Design review of the part shown in the three views and the two pictorial views. Dimensions are in mm from the part's minimum x, y and z. Coordinates: 2 decimals unless noted, no trailing zeros. Order: outer loops, then holes, each group sorted by start corner. A loop starts at its lowest first (then second) coordinate and runs counter-clockwise, first axis right, second up. Notation, with made-up numbers: (-5, 81) -> (48, 81) arc R24 ccw to (48, 120) -> close; hole circle Ø5 at (5.25, 64.25). An arc over 180 degrees is marked (long way). Write item = value, one per line. Start each with the question number.
1) Draft analysis for pull direction Z (two halves, no side actions). For the marked faces 1, 2 and 3, state which applies: +Z half, -Z half, draft (parallel to the pull), parting line (faces both ways), or undercut.
2) Insertion check: pin 1 Ø8 at (x, z) = (19.05, 12.7) entering from +Y. The pin has a flat end and moves straight along its axis. Give the tip position at first contact, or say it passes through.
3) Wall thickness on probe 1 along X at (y, z) = (6.35, 5.5); probe 2 along Y at (x, z) = (44.45, 11.5); probe 3 along Z at (x, y) = (31.75, 3.5): over which ranges is each line inside the solid? List them lowest first. Write a range as [from, to].
4) Consider section C-C on x = 19.05. Give the boundary of the cut face in (y, z), and give its area (3 significant figures).
5) Consider section B-B on z = 12.7. State how many separate pieces and enclosed holes the cut face has.
6) Consider section A-A on y = 6.35. Give the boundary of the cut face in (x, z), and give its area (3 significant figures).
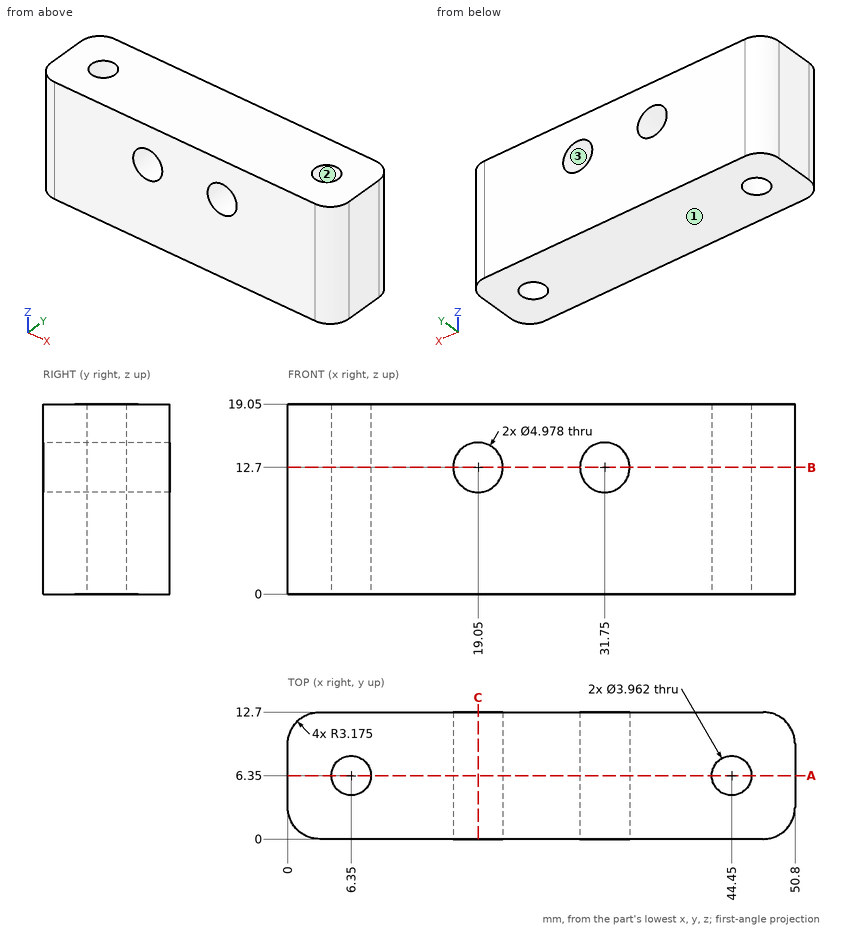
Answer sheet:
q1.face_1 = -Z half
q1.face_2 = draft
q1.face_3 = undercut
q2.pin_1 = 12.7
q3.probe_1 = [0, 4.37], [8.33, 42.47], [46.43, 50.8]
q3.probe_2 = [0, 4.37], [8.33, 12.7]
q3.probe_3 = [0, 10.21], [15.19, 19.05]
q4.outline = (0, 0) -> (12.7, 0) -> (12.7, 10.21) -> (0, 10.21) -> close; (0, 15.19) -> (12.7, 15.19) -> (12.7, 19.05) -> (0, 19.05) -> close
q4.area = 179 mm2
q5.separate_pieces = 3
q5.enclosed_holes = 2
q6.outline = (0, 0) -> (4.37, 0) -> (4.37, 19.05) -> (0, 19.05) -> close; (8.33, 0) -> (42.47, 0) -> (42.47, 19.05) -> (8.33, 19.05) -> close; (46.43, 0) -> (50.8, 0) -> (50.8, 19.05) -> (46.43, 19.05) -> close; hole circle Ø4.98 at (19.05, 12.7); hole circle Ø4.98 at (31.75, 12.7)
q6.area = 778 mm2
